from build123d import *

# Parameters (mm, degrees)
SKETCH_1_W          = 176
SKETCH_1_H          = 89
EXTRUDE_1_DEPTH     = 3
SKETCH_2_R          = 2.025
CUT_EXTRUDE_1_DEPTH = 4
CUT_EXTRUDE_2_DEPTH = 4
SKETCH_4_W          = 116
SKETCH_4_H          = 40
CUT_EXTRUDE_3_DEPTH = 4
SKETCH_5_W          = 92
SKETCH_5_H          = 16
CUT_EXTRUDE_4_DEPTH = 4
CUT_EXTRUDE_5_DEPTH = 24
EXTRUDE_2_DEPTH     = 3
FILLET_1_R          = 2
FILLET_2_R          = 3
SKETCH_8_R          = 7.5
CUT_EXTRUDE_6_DEPTH = 3


with BuildPart() as part:
    # 草图1 → 凸台-拉伸1 (new body)
    with BuildSketch(Plane.XY):
        Rectangle(SKETCH_1_W, SKETCH_1_H)
    extrude(amount=EXTRUDE_1_DEPTH)

    # 草图2 → 切除-拉伸1 (cut)
    with BuildSketch(Plane(origin=(0, 0, 0), x_dir=(-1, 0, 0), z_dir=(0, 0, -1))):
        with Locations((-83.5, 40.2)):
            Circle(SKETCH_2_R)
        with Locations((83.5, 40.2)):
            Circle(SKETCH_2_R)
        with Locations((51, -40.5)):
            Circle(SKETCH_2_R)
        with Locations((-51, -40.5)):
            Circle(SKETCH_2_R)
    extrude(amount=-CUT_EXTRUDE_1_DEPTH, mode=Mode.SUBTRACT)

    # 草图3 → 切除-拉伸2 (cut)
    with BuildSketch(Plane(origin=(0, 0, 0), x_dir=(-1, 0, 0), z_dir=(0, 0, -1))):
        Polygon((88, -44.5), (88, 36.2), (55, -44.5), align=None)
        Polygon((-88, 36.2), (-55, -44.5), (-88, -44.5), align=None)
    extrude(amount=-CUT_EXTRUDE_2_DEPTH, mode=Mode.SUBTRACT)

    # 草图4 → 切除-拉伸3 (cut)
    with BuildSketch(Plane(origin=(0, 0, 0), x_dir=(-1, 0, 0), z_dir=(0, 0, -1))):
        with Locations((0, 44.5)):
            Rectangle(SKETCH_4_W, SKETCH_4_H)
    extrude(amount=-CUT_EXTRUDE_3_DEPTH, mode=Mode.SUBTRACT)

    # 草图5 → 切除-拉伸4 (cut)
    with BuildSketch(Plane(origin=(0, 0, 0), x_dir=(-1, 0, 0), z_dir=(0, 0, -1))):
        with Locations((0, -44.5)):
            Rectangle(SKETCH_5_W, SKETCH_5_H)
    extrude(amount=-CUT_EXTRUDE_4_DEPTH, mode=Mode.SUBTRACT)

    # 草图6 → 切除-拉伸5 (cut)
    with BuildSketch(Plane(origin=(0, 0, 0), x_dir=(-1, 0, 0), z_dir=(0, 0, -1))):
        Polygon((-3, 18.5), (-74.279812328, 18.5), (-54.242637607, -30.5), (-3, -30.5), align=None)
        Polygon((74.279812328, 18.5), (3, 18.5), (3, -30.5), (54.242637607, -30.5), align=None)
    extrude(amount=-CUT_EXTRUDE_5_DEPTH, mode=Mode.SUBTRACT)

    # 草图7 → 凸台-拉伸2 (add)
    with BuildSketch(Plane(origin=(0, 0, 0), x_dir=(-1, 0, 0), z_dir=(0, 0, -1))):
        with BuildLine():
            Line((-52.336918942, -31.106824827), (-37.933084046, 14.128069622))
            Line((-37.933084046, 14.128069622), (-4.617416544, -31.676419875))
            ThreePointArc((-4.617416544, -31.676419875), (-1.823580125, -32.117416544), (-1.382583456, -29.323580125))
            Line((-1.382583456, -29.323580125), (-39.346728283, 22.871930378))
            Line((-39.346728283, 22.871930378), (-56.148356272, -29.893175173))
            ThreePointArc((-56.148356272, -29.893175173), (-54.849462434, -32.405718665), (-52.336918942, -31.106824827))
        make_face()
        with BuildLine():
            Line((4.617416544, -31.676419875), (37.933084046, 14.128069622))
            Line((37.933084046, 14.128069622), (52.336918942, -31.106824827))
            ThreePointArc((52.336918942, -31.106824827), (54.849462434, -32.405718665), (56.148356272, -29.893175173))
            Line((56.148356272, -29.893175173), (39.346728283, 22.871930378))
            Line((39.346728283, 22.871930378), (1.382583456, -29.323580125))
            ThreePointArc((1.382583456, -29.323580125), (1.823580125, -32.117416544), (4.617416544, -31.676419875))
        make_face()
    extrude(amount=-EXTRUDE_2_DEPTH)

    # 圆角1
    fillet_1_edges = [part.edges().sort_by_distance(p)[0] for p in [
        (3, 18.5, 1.5),
        (74.279812328, 18.5, 1.5),
        (-3, 18.5, 1.5),
        (-74.279812328, 18.5, 1.5),
        (36.166826478, 18.5, 1.5),
        (40.738851866, 18.5, 1.5),
        (52.143691905, -30.5, 1.5),
        (5.473079686, -30.5, 1.5),
        (37.933084046, 14.128069622, 1.5),
        (55.422689585, -27.614236527, 1.5),
        (3, -27.099853432, 1.5),
        (-3, -27.099853432, 1.5),
        (-5.473079686, -30.5, 1.5),
        (-52.143691905, -30.5, 1.5),
        (-55.422689585, -27.614236527, 1.5),
        (-40.738851866, 18.5, 1.5),
        (-37.933084046, 14.128069622, 1.5),
        (-36.166826478, 18.5, 1.5),
    ]]
    fillet(fillet_1_edges, radius=FILLET_1_R)

    # 圆角2
    fillet_2_edges = [part.edges().sort_by_distance(p)[0] for p in [
        (88, 36.2, 1.5),
        (55, -44.5, 1.5),
        (-55, -44.5, 1.5),
        (-88, 36.2, 1.5),
        (-58, 44.5, 1.5),
        (-58, 24.5, 1.5),
        (58, 44.5, 1.5),
        (58, 24.5, 1.5),
        (-88, 44.5, 1.5),
        (88, 44.5, 1.5),
        (-46, -44.5, 1.5),
        (-46, -36.5, 1.5),
        (46, -44.5, 1.5),
        (46, -36.5, 1.5),
    ]]
    fillet(fillet_2_edges, radius=FILLET_2_R)

    # 草图8 → 切除-拉伸6 (cut)
    with BuildSketch(Plane.XY.offset(3)):
        with Locations((-70.5, 32)):
            Circle(SKETCH_8_R)
        with Locations(Location((70.5, 32, 0), (0, 0, 180))):
            Circle(SKETCH_8_R)
    extrude(amount=-CUT_EXTRUDE_6_DEPTH, mode=Mode.SUBTRACT)


solid = part.part
Part model, mm, in its own coordinate system. A direction names the side the tool comes from. Coordinates: 2 decimals unless noted, no trailing zeros. Loops run counter-clockwise (first coordinate to the right, second up) from the corner with the lowest first, then second, coordinate; pieces in that order, holes last. Notation, with made-up numbers: (54.25, -30) - (66.25, -30) arc R23 ccw to (66.25, -7) - close; hole circle Ø2 at (29.5, 83). An arc over 180 degrees is marked (long way). Write each question's results on one line, items separated by ' | '. Start each with the question number.
Q1. Which spindle directions (+Z, -Z, +X, -X, +Y, -Y) get a long thin tool onto all of the face, cutting with end or side? Do faces 4 (the flat face through (0, 4, 3)), 5 (the cylindrical face through (4.415, -22.863, 1.479)), 6 (the cylindrical face through (-57.1, 25.36, 1.52)), 7 (the flat face through (1, -36.5, 1)). Say none if no direction does.
Q2. Slice it at A-A on y = 32. Give the cut face in (x, z), and give its area (3 significant figures).
Q3. Slice it at B-B on y = 3. Give the cut face in (x, z).
Q4. Slice it at D-D on y = 20.5. Give the cut face in (x, z).
Q5. Drop flat-ended pins along their axis: pin 1 Ø1.5 at (x, z) = (20, 1.5) entering from -Y; pin 2 Ø0.6 at (y, z) = (-40.5, 1.5) entering from +X; pin 3 Ø0.9 at (x, z) = (-24, 1.5) entering from +Y. Give the stop position or say it passes through.
Q6. Two-plate mould, pull along Y, no slides. Class faces 1 (the cylindrical face through (-46.9, -43.64, 1.52)), 2 (the flat face through (30, -30.5, 1)), 3 (the flat face through (-58, 34, 1)): +Y half, -Y half, draft (parallel to the pull), parting line (faces both ways), or undercut.
Q7. Slice it at C-C on z = 2.5. Give the number of separate pieces and of enclosed holes in the cut face, and give its area (3 significant figures).
Q8. Probe line 1 along X through (y, z) = (37.5, 0.5); line 2 along Y through (x, z) = (-70.5, 1.35); line 3 along X through (y, z) = (34, 1.15). List the from-to ranges inside material, lowest first.
Answer:
1) face 4: +Z, +X, -X, +Y, -Y | face 5: +Z, -Z | face 6: +Z, -Z, +Y | face 7: +Z, -Z, -Y
2) outline: (-86.28, 0) - (-78, 0) - (-78, 3) - (-86.28, 3) - close; (-63, 0) - (-58, 0) - (-58, 3) - (-63, 3) - close; (58, 0) - (63, 0) - (63, 3) - (58, 3) - close; (78, 0) - (86.28, 0) - (86.28, 3) - (78, 3) - close | area: 79.7 mm2
3) outline: (-74.42, 0) - (-67.94, 0) - (-67.94, 3) - (-74.42, 3) - close; (-45.67, 0) - (-41.48, 0) - (-41.48, 3) - (-45.67, 3) - close; (-29.84, 0) - (-24.89, 0) - (-24.89, 3) - (-29.84, 3) - close; (-3, 0) - (3, 0) - (3, 3) - (-3, 3) - close; (24.89, 0) - (29.84, 0) - (29.84, 3) - (24.89, 3) - close; (41.48, 0) - (45.67, 0) - (45.67, 3) - (41.48, 3) - close; (67.94, 0) - (74.42, 0) - (74.42, 3) - (67.94, 3) - close
4) outline: (-81.58, 0) - (81.58, 0) - (81.58, 3) - (-81.58, 3) - close
5) pin 1: stops at y = -36.5 | pin 2: stops at x = 56.76 | pin 3: stops at y = 24.5
6) face 1: -Y half | face 2: undercut | face 3: draft
7) separate pieces: 1 | enclosed holes: 12 | area: 4,450 mm2
8) line 1: x = -88 to -75.6, -65.4 to -58, 58 to 65.4, 75.6 to 88 | line 2: y = -6.6 to 9.26, 18.5 to 24.5, 39.5 to 44.5 | line 3: x = -87.1 to -77.73, -63.27 to -58, 58 to 63.27, 77.73 to 87.1
